For this review, take the finished solid that the model builds, in its own axes (mm). Face numbers are marked on the shaded views. A direction names the side the tool comes from. Round coordinates to 2 decimals unless told otherwise and drop trailing zeros. Order: outer loops, then holes, each group sorted by start corner. A loop starts at its lowest first (then second) coordinate and runs counter-clockwise, first axis right, second up. Notation, with made-up numbers: (48, 68) - (99, 68) arc R21 ccw to (99, 100) - close; hole circle Ø11 at (-4, -1.75). An arc over 180 degrees is marked (long way). Write each question's results on one line, items separated by ' | '. Start each with the question number.
(1) Insertion check: pin 1 Ø5.5 at (x, y) = (0, 0) entering from -Z; pin 2 Ø1 at (y, z) = (1, 16) entering from +X; pin 3 Ø3 at (x, z) = (-5.5, 19) entering from +Y. Each pin has a flat end and moves straight along its axis. Give the tip position at first contact, or say it passes through.
(2) Draft analysis for pull direction Y (two halves, no side actions). For the marked faces 1, 2, 3 and 4, state which applies: pulls with the +Y half, pulls with the -Y half, needs draft (parallel to the pull), parting line crosses it, or undercut.
(3) Take a section at B-B, the plane z = 11.5. Give the boundary of the cut face in (x, y).
(4) Take a section at D-D, the plane z = 4.5. Give the boundary of the cut face in (x, y).
(5) For L1, parallel to Y at x = 0, z = 12.75; L2, parallel to Z at x = 1, y = -13, list the stretches that pass through material, from the lowest coordinate up. Write a range as from..to.
(6) For the marked faces 5 and 6, list the 3-axis set-ups (+Z, -Z, +X, -X, +Y, -Y) from which the entire face can be reached by the end or side of a thin tool; tool diameter is ignored.
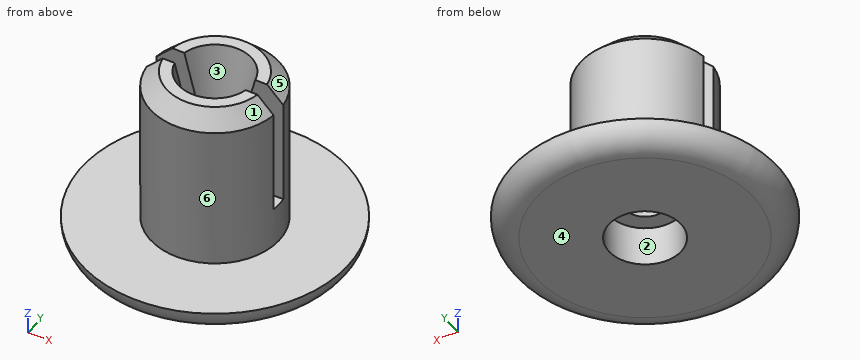
```python
from build123d import *

# Parameters (mm, degrees)
F0_R      = 16.5
F1_DEPTH  = 3
F2_R      = 8
F3_DEPTH  = 20
F4_R      = 2.55
F5_DEPTH  = 25
F6_R      = 4.5
F7_DEPTH  = 5
F8_W      = 17.7715833097
F8_H      = 2
F9_DEPTH  = 15
F10_R     = 2.99999
F11_SIZE  = 2
F12_SIZE2 = 2
F12_SIZE  = 8


# Not quite as in the source:
# - a fillet or chamfer is up to 0.001 mm smaller than in the source, because OpenCascade refuses the exact size


with BuildPart() as f1:
    # F0 (on Top) → F1 (new body)
    with BuildSketch(Plane.XY):
        Circle(F0_R)
    extrude(amount=F1_DEPTH)

    # F2 (on face) → F3 (join)
    with BuildSketch(Plane.XY.offset(3)):
        Circle(F2_R)
    extrude(amount=F3_DEPTH)

    # F4 (on face) → F5 (cut)
    with BuildSketch(Plane(origin=(0, 0, 0), x_dir=(1, 0, 0), z_dir=(0, 0, -1))):
        Circle(F4_R)
    extrude(amount=-F5_DEPTH, mode=Mode.SUBTRACT)

    # F6 (on face) → F7 (cut)
    with BuildSketch(Plane(origin=(0, 0, 0), x_dir=(1, 0, 0), z_dir=(0, 0, -1))):
        Circle(F6_R)
    extrude(amount=-F7_DEPTH, mode=Mode.SUBTRACT)

    # F8 (on face) → F9 (cut)
    with BuildSketch(Plane.XY.offset(23)):
        Rectangle(F8_W, F8_H)
    extrude(amount=-F9_DEPTH, mode=Mode.SUBTRACT)

    # F10 (radius 3 in the source; OpenCascade refuses exactly that, so slightly less here)
    f10_edges = [f1.edges().sort_by_distance(p)[0] for p in [
        (-16.5, 0, 0),
    ]]
    fillet(f10_edges, radius=F10_R)

    # F11
    f11_edges = [f1.edges().sort_by_distance(p)[0] for p in [
        (0, 8, 23),
        (0, -8, 23),
    ]]
    chamfer(f11_edges, length=F11_SIZE)

    # F12
    f12_edges = [f1.edges().sort_by_distance(p)[0] for p in [
        (0, 2.55, 23),
        (0, -2.55, 23),
    ]]
    f12_side = f1.faces().sort_by_distance((2.498413, 0.510324, 7.806088))[0]
    chamfer(f12_edges, length=F12_SIZE, length2=F12_SIZE2, reference=f12_side)


solid = f1.part
```
Results below:
1) pin 1: stops at z = 5 | pin 2: stops at x = 7.94 | pin 3: stops at y = 6.93
2) face 1: pulls with the -Y half | face 2: undercut | face 3: undercut | face 4: needs draft
3) outline: (-7.94, -1) arc R8 ccw to (7.94, -1) - (2.35, -1) arc R2.55 cw to (-2.35, -1) - close; (-7.94, 1) - (-2.35, 1) arc R2.55 cw to (2.35, 1) - (7.94, 1) arc R8 ccw to start
4) outline: circle Ø16 at (0, 0); hole circle Ø9 at (0, 0)
5) L1: y = -8..-2.55, 2.55..8 | L2: z = 0..3
6) face 5: +Z, +Y | face 6: +Z
